```python
from build123d import *

# Parameters (mm, degrees)
CYLINDER011_R     = 15
CYLINDER011_DEPTH = 2
SKETCH009_R       = 1.6
PAD012_DEPTH      = 5


with BuildPart() as cilindro011:
    # Cylinder011 → Cylinder011 (new body)
    with BuildSketch(Plane(origin=(206.5, 0, -27.5), x_dir=(1, 0, 0), z_dir=(0, 0, 1))):
        Circle(CYLINDER011_R)
    extrude(amount=CYLINDER011_DEPTH)


with BuildPart() as cut007:
    # Sketch009 → Pad012 (new body)
    with BuildSketch(Plane.XY.offset(-27.5)):
        with BuildLine():
            ThreePointArc((201.551358, -0.714804), (207.214804, -4.948642), (211.448642, 0.714804))
            Line((211.448642, 0.714804), (204.948642, 45.714804))
            ThreePointArc((204.948642, 45.714804), (199.285196, 49.948642), (195.051358, 44.285196))
            Line((201.551358, -0.714804), (195.051358, 44.285196))
        make_face()
        with Locations((200, 45)):
            Circle(SKETCH009_R, mode=Mode.SUBTRACT)
        with Locations((206.5, 0)):
            Circle(SKETCH009_R, mode=Mode.SUBTRACT)
    extrude(amount=PAD012_DEPTH)

    # Cut007: cut Cilindro011
    add(cilindro011.part, mode=Mode.SUBTRACT)


solid = cut007.part
```
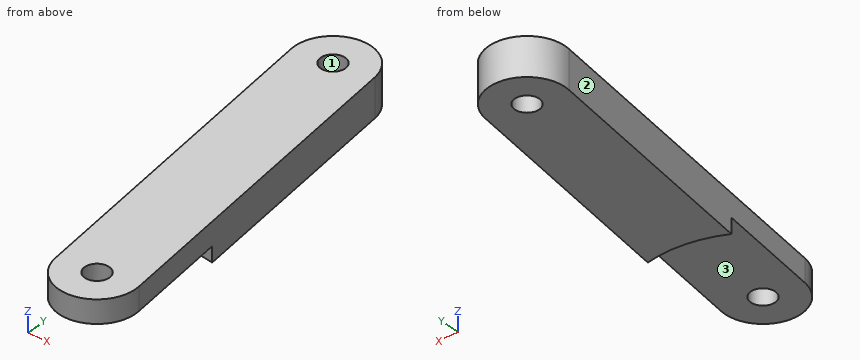
Input: part model. Units: mm. Frame: model coordinates. Face numbers are marked on the shaded views. Give positions to 0.01 mm unless a question says otherwise; leave off trailing zeros. Write each loop counter-clockwise with the first axis right and the second up, starting at its lowest first coordinate (ties: lowest second). Pieces come first, ordered by that corner, then holes. Notation, with made-up numbers: (34, 49.25) - (40, 49.25) arc R19 ccw to (40, 79.25) - close; hole circle Ø4 at (2.25, -14.75). An arc over 180 degrees is marked (long way). Write item = value, one per line. Start each with the question number.
1. Section query B-B, the plane y = 45. Output: boundary loops of the cut face in (x, z).
2. Mould query, pull axis Y, two halves, no side actions, for the marked faces 1, 2 and 3. Classes: released by +Y, released by -Y, zero draft, split by the parting line, or undercut.
3. Section query A-A, the plane x = 200. Output: boundary loops of the cut face in (y, z), then the cut area to 3 significant figures.
4. Section query D-D, the plane x = 206.5. Output: boundary loops of the cut face in (y, z), then the cut area to 3 significant figures.
5. Section query C-C, the plane z = -24.4. Output: boundary loops of the cut face in (x, y), then the cut area to 3 significant figures.
6. First-contact query: pin 1 Ø3.5 at (x, y) = (206.5, 0) entering from -Z; pin 2 Ø6 at (x, y) = (197, 28) entering from -Z; pin 3 Ø1 at (y, z) = (43.5, -23.5) entering from +X. Flat tips, straight axial feed; report the tip coordinate or a pass-through.
7. Ray query, L1, parallel to Z at x = 206.5, y = 3; L2, parallel to X at y = 0, z = -23.2; L3, parallel to X at y = 47, z = -23.3. Return the intervals inside material, ascending.
Check sheet entries:
q1.outline = (195, -27.5) - (198.4, -27.5) - (198.4, -22.5) - (195, -22.5) - close; (201.6, -27.5) - (205.05, -27.5) - (205.05, -22.5) - (201.6, -22.5) - close
q2.face_1 = undercut
q2.face_2 = released by -Y
q2.face_3 = zero draft
q3.outline = (10.03, -25.5) - (13.52, -25.5) - (13.52, -27.5) - (43.4, -27.5) - (43.4, -22.5) - (10.03, -22.5) - close; (46.6, -27.5) - (50, -27.5) - (50, -22.5) - (46.6, -22.5) - close
q3.area = 177 mm2
q4.outline = (-5, -25.5) - (-1.6, -25.5) - (-1.6, -22.5) - (-5, -22.5) - close; (1.6, -25.5) - (15, -25.5) - (15, -27.5) - (34.97, -27.5) - (34.97, -22.5) - (1.6, -22.5) - close
q4.area = 150 mm2
q5.outline = (195.05, 44.29) - (201.55, -0.71) arc R5 ccw to (211.45, 0.71) - (204.95, 45.71) arc R5 ccw to start; hole circle Ø3.2 at (200, 45); hole circle Ø3.2 at (206.5, 0)
q5.area = 517 mm2
q6.pin_1 = -25.5
q6.pin_2 = -27.5
q6.pin_3 = 205.34
q7.L1 = -25.5 to -22.5
q7.L2 = 201.45 to 204.9, 208.1 to 211.5
q7.L3 = 195.42 to 204.58
